Verification items for the finished model (mm, model axes). Face numbers are marked on the shaded views. A direction names the side the tool comes from. Coordinates: 2 decimals unless noted, no trailing zeros. Write each loop counter-clockwise with the first axis right and the second up, starting at its lowest first coordinate (ties: lowest second). Pieces come first, ordered by that corner, then holes.
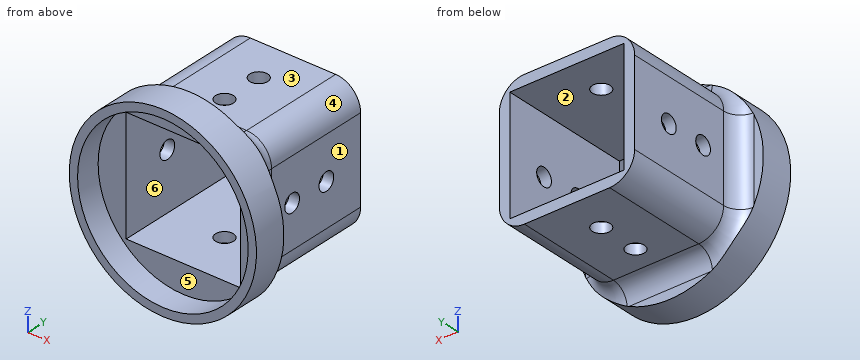
```python
from build123d import *

# Parameters (mm, degrees)
SKETCH_1_R          = 22.5
SKETCH_1_R_2        = 20.5
EXTRUDE_1_DEPTH     = 6
SKETCH_2_R          = 22.5
EXTRUDE_2_DEPTH     = 2
SKETCH_3_W          = 26.5
SKETCH_3_H          = 26.5
SKETCH_3_W_2        = 20.5
SKETCH_3_H_2        = 20.5
EXTRUDE_3_DEPTH     = 30
SKETCH_4_R          = 2.15
CUT_EXTRUDE_1_DEPTH = 30
SKETCH_5_R          = 2.15
CUT_EXTRUDE_2_DEPTH = 30
FILLET_1_R          = 3
SKETCH_7_W          = 26.5
SKETCH_7_H          = 26.5
EXTRUDE_4_DEPTH     = 30
SKETCH_8_W          = 27.5
SKETCH_8_H          = 27.5
CUT_EXTRUDE_4_DEPTH = 50.563091106
FILLET_2_R          = 4
SKETCH_9_R          = 2.15
CUT_EXTRUDE_5_DEPTH = 59.752127725
SKETCH_10_R         = 2.15
CUT_EXTRUDE_6_DEPTH = 59.752127725


with BuildPart() as part:
    # 草图1 → 凸台-拉伸1 (new body)
    with BuildSketch(Plane(origin=(0, 0, 0), x_dir=(1, 0, 0), z_dir=(0, 1, 0))):
        with Locations(Location((0, 0, 0), (0, 0, 270))):
            Circle(SKETCH_1_R)
        with Locations(Location((0, 0, 0), (0, 0, 270))):
            Circle(SKETCH_1_R_2, mode=Mode.SUBTRACT)
    extrude(amount=EXTRUDE_1_DEPTH)

    # 草图2 → 凸台-拉伸2 (add)
    with BuildSketch(Plane(origin=(0, 6, 0), x_dir=(1, 0, 0), z_dir=(0, 1, 0))):
        with Locations(Location((0, 0, 0), (0, 0, 270))):
            Circle(SKETCH_2_R)
    extrude(amount=EXTRUDE_2_DEPTH)

    # 草图3 → 凸台-拉伸3 (add)
    with BuildSketch(Plane(origin=(0, 8, 0), x_dir=(1, 0, 0), z_dir=(0, 1, 0))):
        Rectangle(SKETCH_3_W, SKETCH_3_H)
        Rectangle(SKETCH_3_W_2, SKETCH_3_H_2, mode=Mode.SUBTRACT)
    extrude(amount=EXTRUDE_3_DEPTH)

    # 草图4 → 切除-拉伸1 (cut)
    with BuildSketch(Plane.XY.offset(13.25)):
        with Locations((0, 28)):
            Circle(SKETCH_4_R)
        with Locations((0, 18)):
            Circle(SKETCH_4_R)
    extrude(amount=-CUT_EXTRUDE_1_DEPTH, mode=Mode.SUBTRACT)

    # 草图5 → 切除-拉伸2 (cut)
    with BuildSketch(Plane(origin=(13.25, 0, 0), x_dir=(0, 0, -1), z_dir=(1, 0, 0))):
        with Locations((0, 28)):
            Circle(SKETCH_5_R)
        with Locations((0, 18)):
            Circle(SKETCH_5_R)
    extrude(amount=-CUT_EXTRUDE_2_DEPTH, mode=Mode.SUBTRACT)

    # 圆角1
    fillet_1_edges = [part.edges().sort_by_distance(p)[0] for p in [
        (-13.25, 23, -13.25),
        (-13.25, 23, 13.25),
        (13.25, 23, 13.25),
        (13.25, 23, -13.25),
    ]]
    fillet(fillet_1_edges, radius=FILLET_1_R)

    # 草图7 → 凸台-拉伸4 (add)
    with BuildSketch(Plane(origin=(0, 38, 0), x_dir=(1, 0, 0), z_dir=(0, 1, 0))):
        with BuildLine():
            Line((-16.25, 10.25), (-16.25, -10.25))
            ThreePointArc((-16.25, -10.25), (-14.492640687, -14.492640687), (-10.25, -16.25))
            Line((-10.25, -16.25), (10.25, -16.25))
            ThreePointArc((10.25, -16.25), (14.492640687, -14.492640687), (16.25, -10.25))
            Line((16.25, -10.25), (16.25, 10.25))
            ThreePointArc((16.25, 10.25), (14.492640687, 14.492640687), (10.25, 16.25))
            Line((10.25, 16.25), (-10.25, 16.25))
            ThreePointArc((-10.25, 16.25), (-14.492640687, 14.492640687), (-16.25, 10.25))
        make_face()
        Rectangle(SKETCH_7_W, SKETCH_7_H, mode=Mode.SUBTRACT)
    extrude(amount=-EXTRUDE_4_DEPTH)

    # 草图8 → 切除-拉伸4 (cut, through all)
    with BuildSketch(Plane(origin=(0, 38, 0), x_dir=(1, 0, 0), z_dir=(0, 1, 0))):
        Rectangle(SKETCH_8_W, SKETCH_8_H)
    extrude(amount=-CUT_EXTRUDE_4_DEPTH, mode=Mode.SUBTRACT)

    # 圆角2
    # the kernel refuses this fillet: 4 mm, written as the material it adds along each edge
    with BuildSketch(Plane(origin=(-10.25, 8, -10.25), x_dir=(0, 0, -1), z_dir=(1, 0, 0))) as fillet_2_piece_1_section:
        with BuildLine():
            CenterArc((6 + FILLET_2_R, FILLET_2_R), FILLET_2_R, 180, 90)
            Line((6, FILLET_2_R), (6, 0))
            Line((6, 0), (6 + FILLET_2_R, 0))
        make_face()
    fillet_2_piece_1 = revolve(axis=Axis((-10.25, 8, -10.25), (0, 1, 0)), revolution_arc=90, mode=Mode.PRIVATE)
    fillet_2_piece_1 = fillet_2_piece_1 & Plane(origin=(0, 8.919609383, 0), x_dir=(0, 0, 1), z_dir=(0, -1, 0)) * Cylinder(22.5, 40, mode=Mode.PRIVATE)
    add(fillet_2_piece_1)
    with BuildSketch(Plane(origin=(10.25, 8, -16.25), x_dir=(0, 0, -1), z_dir=(-1, 0, 0))) as fillet_2_piece_2_section:
        with BuildLine():
            CenterArc((FILLET_2_R, -FILLET_2_R), FILLET_2_R, 90, 90)
            Line((0, -FILLET_2_R), (0, 0))
            Line((0, 0), (FILLET_2_R, 0))
        make_face()
    fillet_2_piece_2 = extrude(amount=20.5, mode=Mode.PRIVATE)
    fillet_2_piece_2 = fillet_2_piece_2 & Plane(origin=(0, 8.90566888, 0), x_dir=(0, 0, 1), z_dir=(0, -1, 0)) * Cylinder(22.5, 57, mode=Mode.PRIVATE)
    add(fillet_2_piece_2)
    with BuildSketch(Plane(origin=(10.25, 8, -10.25), x_dir=(1, 0, 0), z_dir=(0, 0, 1))) as fillet_2_piece_3_section:
        with BuildLine():
            CenterArc((6 + FILLET_2_R, FILLET_2_R), FILLET_2_R, 180, 90)
            Line((6, FILLET_2_R), (6, 0))
            Line((6, 0), (6 + FILLET_2_R, 0))
        make_face()
    fillet_2_piece_3 = revolve(axis=Axis((10.25, 8, -10.25), (0, 1, 0)), revolution_arc=90, mode=Mode.PRIVATE)
    fillet_2_piece_3 = fillet_2_piece_3 & Plane(origin=(0, 8.919609383, 0), x_dir=(0, 0, 1), z_dir=(0, -1, 0)) * Cylinder(22.5, 40, mode=Mode.PRIVATE)
    add(fillet_2_piece_3)
    with BuildSketch(Plane(origin=(16.25, 8, 10.25), x_dir=(1, 0, 0), z_dir=(0, 0, -1))) as fillet_2_piece_4_section:
        with BuildLine():
            CenterArc((FILLET_2_R, -FILLET_2_R), FILLET_2_R, 90, 90)
            Line((0, -FILLET_2_R), (0, 0))
            Line((0, 0), (FILLET_2_R, 0))
        make_face()
    fillet_2_piece_4 = extrude(amount=20.5, mode=Mode.PRIVATE)
    fillet_2_piece_4 = fillet_2_piece_4 & Plane(origin=(0, 8.90566888, 0), x_dir=(0, 0, 1), z_dir=(0, -1, 0)) * Cylinder(22.5, 57, mode=Mode.PRIVATE)
    add(fillet_2_piece_4)
    with BuildSketch(Plane(origin=(10.25, 8, 10.25), x_dir=(0, 0, 1), z_dir=(-1, 0, 0))) as fillet_2_piece_5_section:
        with BuildLine():
            CenterArc((6 + FILLET_2_R, FILLET_2_R), FILLET_2_R, 180, 90)
            Line((6, FILLET_2_R), (6, 0))
            Line((6, 0), (6 + FILLET_2_R, 0))
        make_face()
    fillet_2_piece_5 = revolve(axis=Axis((10.25, 8, 10.25), (0, 1, 0)), revolution_arc=90, mode=Mode.PRIVATE)
    fillet_2_piece_5 = fillet_2_piece_5 & Plane(origin=(0, 8.919609383, 0), x_dir=(0, 0, 1), z_dir=(0, -1, 0)) * Cylinder(22.5, 40, mode=Mode.PRIVATE)
    add(fillet_2_piece_5)
    with BuildSketch(Plane(origin=(-10.25, 8, 16.25), x_dir=(0, 0, 1), z_dir=(1, 0, 0))) as fillet_2_piece_6_section:
        with BuildLine():
            CenterArc((FILLET_2_R, -FILLET_2_R), FILLET_2_R, 90, 90)
            Line((0, -FILLET_2_R), (0, 0))
            Line((0, 0), (FILLET_2_R, 0))
        make_face()
    fillet_2_piece_6 = extrude(amount=20.5, mode=Mode.PRIVATE)
    fillet_2_piece_6 = fillet_2_piece_6 & Plane(origin=(0, 8.90566888, 0), x_dir=(0, 0, 1), z_dir=(0, -1, 0)) * Cylinder(22.5, 57, mode=Mode.PRIVATE)
    add(fillet_2_piece_6)
    with BuildSketch(Plane(origin=(-10.25, 8, 10.25), x_dir=(-1, 0, 0), z_dir=(0, 0, -1))) as fillet_2_piece_7_section:
        with BuildLine():
            CenterArc((6 + FILLET_2_R, FILLET_2_R), FILLET_2_R, 180, 90)
            Line((6, FILLET_2_R), (6, 0))
            Line((6, 0), (6 + FILLET_2_R, 0))
        make_face()
    fillet_2_piece_7 = revolve(axis=Axis((-10.25, 8, 10.25), (0, 1, 0)), revolution_arc=90, mode=Mode.PRIVATE)
    fillet_2_piece_7 = fillet_2_piece_7 & Plane(origin=(0, 8.919609383, 0), x_dir=(0, 0, 1), z_dir=(0, -1, 0)) * Cylinder(22.5, 40, mode=Mode.PRIVATE)
    add(fillet_2_piece_7)
    with BuildSketch(Plane(origin=(-16.25, 8, -10.25), x_dir=(-1, 0, 0), z_dir=(0, 0, 1))) as fillet_2_piece_8_section:
        with BuildLine():
            CenterArc((FILLET_2_R, -FILLET_2_R), FILLET_2_R, 90, 90)
            Line((0, -FILLET_2_R), (0, 0))
            Line((0, 0), (FILLET_2_R, 0))
        make_face()
    fillet_2_piece_8 = extrude(amount=20.5, mode=Mode.PRIVATE)
    fillet_2_piece_8 = fillet_2_piece_8 & Plane(origin=(0, 8.90566888, 0), x_dir=(0, 0, 1), z_dir=(0, -1, 0)) * Cylinder(22.5, 57, mode=Mode.PRIVATE)
    add(fillet_2_piece_8)

    # 草图9 → 切除-拉伸5 (cut, through all)
    with BuildSketch(Plane(origin=(16.25, 0, 0), x_dir=(0, 0, -1), z_dir=(1, 0, 0))):
        with Locations((0, 28)):
            Circle(SKETCH_9_R)
        with Locations((0, 18)):
            Circle(SKETCH_9_R)
    extrude(amount=-CUT_EXTRUDE_5_DEPTH, mode=Mode.SUBTRACT)

    # 草图10 → 切除-拉伸6 (cut, through all)
    with BuildSketch(Plane.XY.offset(16.25)):
        with Locations((0, 28)):
            Circle(SKETCH_10_R)
        with Locations((0, 18)):
            Circle(SKETCH_10_R)
    extrude(amount=-CUT_EXTRUDE_6_DEPTH, mode=Mode.SUBTRACT)


solid = part.part
```
1. Sectioned sample at A-A, the plane z = 0. Give the number of separate pieces and of enclosed holes in the cut face, and give its area (3 significant figures).
2. Sectioned sample at D-D, the plane y = 28. Record the boundary of the cut face in (x, z), and give its area (3 significant figures).
3. Gauge pin test, flat ends, axial feed: P1, Ø8, axis at x = -8, y = 13, coming from the +Z side; P2, Ø2, axis at y = 22, z = 12.5, coming from the -X side; P3, Ø5.5, axis at y = 18, z = 0, coming from the -X side. Record the tip position at first contact, or that the pin passes through.
4. Material ranges on L1, parallel to Y at x = 0, z = 15.65; L2, parallel to Z at x = 6, y = 13, recorded low to high.
5. Tool access check on the marked faces 4, 5 and 6. Record the directions out of +Z, -Z, +X, -X, +Y, -Y that give a thin tool (end or side, any length) a straight path to the whole face; none if there is none.
6. Sectioned sample at C-C, the plane x = -3. Record the boundary of the cut face in (y, z).
7. Sectioned sample at B-B, the plane y = 22.5. Record the boundary of the cut face in (x, z).
8. Draft check along X on the marked faces 1, 2 and 3. Enter one of: pulls with the +X half, pulls with the -X half, needs draft (parallel to the pull), parting line crosses it, or undercut.
Outcome:
1. separate pieces: 6
1. enclosed holes: 0
1. area: 173 mm2
2. outline: (-16.25, -10.25) arc R6 ccw to (-10.25, -16.25) - (-2.15, -16.25) - (-2.15, -13.75) - (-13.75, -13.75) - (-13.75, -2.15) - (-16.25, -2.15) - close; (-16.25, 2.15) - (-13.75, 2.15) - (-13.75, 13.75) - (-2.15, 13.75) - (-2.15, 16.25) - (-10.25, 16.25) arc R6 ccw to (-16.25, 10.25) - close; (2.15, -16.25) - (10.25, -16.25) arc R6 ccw to (16.25, -10.25) - (16.25, -2.15) - (13.75, -2.15) - (13.75, -13.75) - (2.15, -13.75) - close; (2.15, 13.75) - (13.75, 13.75) - (13.75, 2.15) - (16.25, 2.15) - (16.25, 10.25) arc R6 ccw to (10.25, 16.25) - (2.15, 16.25) - close
2. area: 226 mm2
3. P1: stops at z = 17.6
3. P2: stops at x = -16.12
3. P3: stops at x = -16.25
4. L1: y = 6 to 15.85, 20.15 to 25.85, 30.15 to 38
4. L2: z = -16.25 to -13.75, 13.75 to 16.25
5. face 4: +Z, +X, +Y
5. face 5: -Y
5. face 6: +Y, -Y
6. outline: (0, -22.3) - (8, -22.3) - (8, -20.25) arc R4 cw to (12, -16.25) - (38, -16.25) - (38, -13.75) - (6, -13.75) - (6, -20.28) - (0, -20.28) - close; (0, 20.28) - (6, 20.28) - (6, 13.75) - (38, 13.75) - (38, 16.25) - (12, 16.25) arc R4 cw to (8, 20.25) - (8, 22.3) - (0, 22.3) - close
7. outline: (-16.25, -10.25) arc R6 ccw to (-10.25, -16.25) - (10.25, -16.25) arc R6 ccw to (16.25, -10.25) - (16.25, 10.25) arc R6 ccw to (10.25, 16.25) - (-10.25, 16.25) arc R6 ccw to (-16.25, 10.25) - close; hole (-13.75, -13.75) - (13.75, -13.75) - (13.75, 13.75) - (-13.75, 13.75) - close
8. face 1: pulls with the +X half
8. face 2: undercut
8. face 3: needs draft
